Verification items for the finished model (mm, model axes). Face numbers are marked on the shaded views. Coordinates: 2 decimals unless noted, no trailing zeros. Order: outer loops, then holes, each group sorted by start corner. A loop starts at its lowest first (then second) coordinate and runs counter-clockwise, first axis right, second up. Notation, with made-up numbers: (47, 70) -> (56, 70) arc R32 ccw to (56, 98) -> close; hole circle Ø4 at (-13.5, 74). An arc over 180 degrees is marked (long way). Write item = value, one per line. Start each with the question number.
1. Cross-section at B-B on z = 18. Record the cut outline in (x, y) (3 decimals), plus the area to 3 significant figures.
2. Thickness scan on line 1 along Y through (x, z) = (0, 14.5) (3 decimals); line 2 along X through (y, z) = (0.25, 9.25); line 3 along Z through (x, y) = (3.25, -0.5) (3 decimals). Record the ranges inside material, lowest first. Write a range as from..to.
3. Cross-section at A-A on y = 0. Record the cut outline in (x, z) (3 decimals).
4. Release check for a two-part mould opening along X. For the marked faces 1, 2 and 3 record: +X half, -X half, draft (parallel to the pull), parting line (faces both ways), or undercut.
5. Go/stop test with flat-tipped pins: P1, Ø1, axis at y = 8.5, z = 8.5, coming from the +X side; P2, Ø12, axis at x = 10, z = 5.5, coming from the +Y side; P3, Ø6, axis at y = -4.5, z = 11.5, coming from the -X side. Record where each tip stops, or that it passes through.
Autodesk Inventor part; units mm, degrees
ref_plane "YZ Plane" through (0, 0, 0) normal (1, 0, 0) x (0, 1, 0)
ref_plane "XZ Plane" through (0, 0, 0) normal (0, 1, 0) x (-1, 0, 0)
ref_plane "XY Plane" through (0, 0, 0) normal (0, 0, 1) x (1, 0, 0)
sketch "Sketch1" plane through (0, 0, 0) normal (0, 0, 1) x (1, 0, 0)
  circle A0 centre (0, 0) radius 13.335
  circle A1 centre (0, 0) radius 10.795
  dimension "d0" = 26.67
  dimension "d2" = 21.59
extrude "Extrusion1" add sketch "Sketch1" along normal blind 19.05
sketch "Sketch2" plane through (0, 0, 19.05) normal (0, 0, 1) x (1, 0, 0)
  circle A0 centre (0, 0) radius 13.335
extrude "Extrusion2" add sketch "Sketch2" along normal blind 3.175
fillet "Fillet1" radius 3.175 1 edges at (-13.335, 0, 22.225)
properties part number "Cap" material "PVC-Piping"
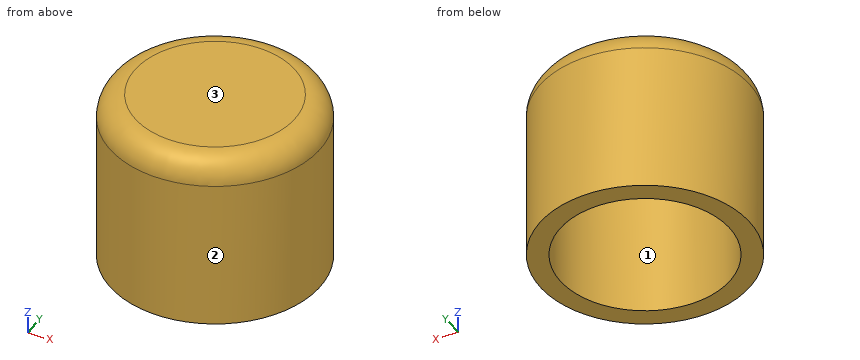
Worked out:
q1.outline = circle Ø26.67 at (0, 0); hole circle Ø21.59 at (0, 0)
q1.area = 193 mm²
q2.line_1 = -13.335..-10.795, 10.795..13.335
q2.line_2 = -13.33..-10.79, 10.79..13.33
q2.line_3 = 19.05..22.225
q3.outline = (-13.335, 0) -> (-10.795, 0) -> (-10.795, 19.05) -> (10.795, 19.05) -> (10.795, 0) -> (13.335, 0) -> (13.335, 19.05) arc R3.175 ccw to (10.16, 22.225) -> (-10.16, 22.225) arc R3.175 ccw to (-13.335, 19.05) -> close
q4.face_1 = undercut
q4.face_2 = parting line
q4.face_3 = draft
q5.P1 = 10.67
q5.P2 = 12.72
q5.P3 = -13.25
